Autodesk Inventor part; units mm, degrees
ref_plane "YZ Plane" through (0, 0, 0) normal (1, 0, 0) x (0, 1, 0)
ref_plane "XZ Plane" through (0, 0, 0) normal (0, 1, 0) x (-1, 0, 0)
ref_plane "XY Plane" through (0, 0, 0) normal (0, 0, 1) x (1, 0, 0)
sketch "Skizze1" plane through (0, 0, 0) normal (0, 0, 1) x (1, 0, 0)
  circle A0 centre (0, 0) radius 9.25
  dimension "d0" = 18.5
extrude "Extrusion1" add sketch "Skizze1" along normal mid plane 69
sketch "Skizze2" plane through (0, 0, 34.5) normal (0, 0, 1) x (1, 0, 0)
  circle A0 centre (0, 0) radius 3.3
  circle A1 centre (0, 0) radius 9.25
  dimension "d3" = 6.6
extrude "Extrusion2" cut sketch "Skizze2" against normal blind 1
sketch "Skizze3" plane through (0, 0, 0) normal (0, 1, 0) x (-1, 0, 0)
  line L0 (9.25, -34.5) -> (9.25, 33.5) construction
  line L1 (9.25, -31.25) -> (9, -31.5)
  line L2 (9, -31.5) -> (9.25, -31.75)
  line L3 (-9.25, -34.5) -> (9.25, -34.5)
  line L4 (9.25, -31.75) -> (9.25, -31.25)
  line L5 (0, -46.714) -> (0, 45.714)
  point P0 (0, 0)
  dimension "d6" = 3
  dimension "d7" = 0.5
revolve "Umdrehung1" cut sketch "Skizze3" angle 360 about axis through (0, 0, -10) along (0, 0, 1)
properties part number "18650" material "Nickel-Kupfer-Legierung 400"
Model file for the job. Use its own axes, mm. A direction names the side the tool comes from. Give positions to 0.01 mm unless a question says otherwise; leave off trailing zeros. Order: outer loops, then holes, each group sorted by start corner. A loop starts at its lowest first (then second) coordinate and runs counter-clockwise, first axis right, second up. Notation, with made-up numbers: (3, 88) - (44, 88) arc R14 ccw to (44, 103) - close; hole circle Ø9 at (-18, 5). An arc over 180 degrees is marked (long way). One line per item, written item: value.
Item 1: Tool access for faces 1 (the cylindrical face through (-2.01, -9.03, -33.11)), 2 (the cylindrical face through (-2.43, 2.23, 34.01)): list every direction of +Z, -Z, +X, -X, +Y, -Y with a clear straight run to the whole face (end or side of a thin tool).
Response values:
face 1: +Z, -Z
face 2: +Z
Item 2: Pin check, flat tips, straight feed: pin 1 Ø4 at (x, z) = (7.5, -27) entering from +Y; pin 2 Ø1.5 at (x, z) = (-4.5, 7) entering from -Y; pin 3 Ø1.5 at (y, z) = (-4.5, 20.5) entering from +X. Stop position of each tip, or through.
Response values:
pin 1: y = 7.44
pin 2: y = -8.46
pin 3: x = 8.46
Item 3: Wall check: line 1 (Z direction, x = 1.5, y = -3.25); line 2 (X direction, y = 0.25, z = -23); line 3 (Y direction, x = 2.75, z = 3). Give the ranges that are in metal, low to high.
Response values:
line 1: -34.5 to 33.5
line 2: -9.25 to 9.25
line 3: -8.83 to 8.83
Item 4: Slice it at A-A (z = 26). List the corners of the cut face in (x, y).
Response values:
outline: circle Ø18.5 at (0, 0)
